Check sheet for the modelled part. Datum: model origin and axes. Units: mm. Face numbers are marked on the shaded views. Coordinates: 2 decimals unless noted, no trailing zeros. Write each loop counter-clockwise with the first axis right and the second up, starting at its lowest first coordinate (ties: lowest second). Pieces come first, ordered by that corner, then holes. Notation, with made-up numbers: M 51.5,-34 L 65.5,-34 A24 ccw 65.5,-6 Z; hole C 64,49 d11. An arc over 180 degrees is marked long. Answer as CSV lines item,"result". Start each with the question number.
1) Section check B-B (x = 0). Record the cut outline in (y, z).
2) Section check C-C (y = 1.5). Record the cut outline in (x, z), and give its area (3 significant figures).
3) Material ranges on L1, parallel to Y at x = 0, z = -19.25; L2, parallel to Y at x = 3, z = -5.5; L3, parallel to X at y = -17.5, z = -10.5, recorded low to high. Write a range as [from, to].
4) Section check D-D (x = -19). Record the cut outline in (y, z).
5) Section check A-A (z = -15.25). Record the cut outline in (x, y).
6) Draft check along X on the marked faces 1, 2 and 3. Enter one of: +X half, -X half, draft (parallel to the pull), parting line (faces both ways), or undercut.
7) Go/stop test with flat-tipped pins: pin 1 Ø6 at (x, z) = (15.5, -4.5) entering from +Y; pin 2 Ø12 at (y, z) = (-17.5, -22) entering from -X; pin 3 Ø1.5 at (y, z) = (-20, -8) entering from +X; pin 4 Ø9 at (x, y) = (0, 20) entering from -Z. Record where each tip stops, or that it passes through.
from build123d import *

# Parameters (mm, degrees)
SKETCH_1_R          = 27.5
EXTRUDE_1_DEPTH     = 25
SKETCH_2_R          = 12.5
SKETCH_2_R_2        = 3.5
CUT_EXTRUDE_1_DEPTH = 25


with BuildPart() as part:
    # 草图1 → 凸台-拉伸1 (new body)
    with BuildSketch(Plane.XY):
        Circle(SKETCH_1_R)
    extrude(amount=-EXTRUDE_1_DEPTH)

    # 草图2 → 切除-拉伸1 (cut)
    with BuildSketch(Plane.XY):
        Circle(SKETCH_2_R)
        with Locations((20, 0)):
            Circle(SKETCH_2_R_2)
        with Locations((0, 20)):
            Circle(SKETCH_2_R_2)
        with Locations((-20, 0)):
            Circle(SKETCH_2_R_2)
        with Locations((0, -20)):
            Circle(SKETCH_2_R_2)
    extrude(amount=-CUT_EXTRUDE_1_DEPTH, mode=Mode.SUBTRACT)


solid = part.part
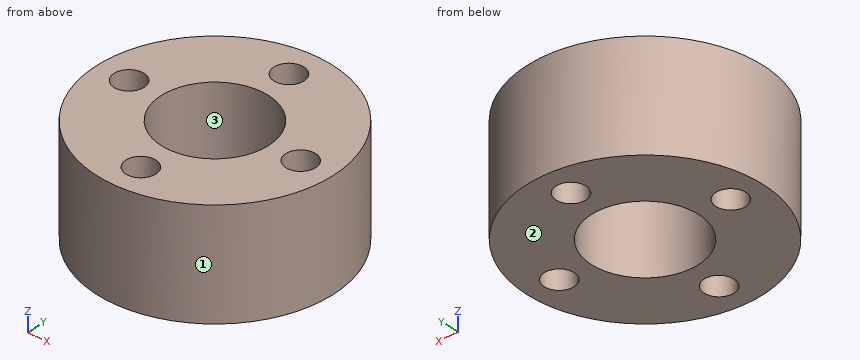
Results found:
1,outline,"M -27.5,-25 L -23.5,-25 L -23.5,0 L -27.5,0 Z; M -16.5,-25 L -12.5,-25 L -12.5,0 L -16.5,0 Z; M 12.5,-25 L 16.5,-25 L 16.5,0 L 12.5,0 Z; M 23.5,-25 L 27.5,-25 L 27.5,0 L 23.5,0 Z"
2,outline,"M -27.46,-25 L -23.16,-25 L -23.16,0 L -27.46,0 Z; M -16.84,-25 L -12.41,-25 L -12.41,0 L -16.84,0 Z; M 12.41,-25 L 16.84,-25 L 16.84,0 L 12.41,0 Z; M 23.16,-25 L 27.46,-25 L 27.46,0 L 23.16,0 Z"
2,area,"436 mm2"
3,L1,"y = [-27.5, -23.5], [-16.5, -12.5], [12.5, 16.5], [23.5, 27.5]"
3,L2,"y = [-27.34, -21.8], [-18.2, -12.13], [12.13, 18.2], [21.8, 27.34]"
3,L3,"x = [-21.21, -2.45], [2.45, 21.21]"
4,outline,"M -19.88,-25 L -3.35,-25 L -3.35,0 L -19.88,0 Z; M 3.35,-25 L 19.88,-25 L 19.88,0 L 3.35,0 Z"
5,outline,"C 0,0 d55; hole C -20,0 d7; hole C 0,0 d25; hole C 0,-20 d7; hole C 0,20 d7; hole C 20,0 d7"
6,face 1,"parting line"
6,face 2,"draft"
6,face 3,"undercut"
7,pin 1,"stops at y = 24.49"
7,pin 2,"stops at x = -24.98"
7,pin 3,"stops at x = 19.64"
7,pin 4,"stops at z = -25"
